Part model, mm, in its own coordinate system. Coordinates: 2 decimals unless noted, no trailing zeros. Loops run counter-clockwise (first coordinate to the right, second up) from the corner with the lowest first, then second, coordinate; pieces in that order, holes last. Notation, with made-up numbers: M 60,73 L 75,73 A6 ccw 75,79 Z; hole C 43.5,-20 d8. An arc over 180 degrees is marked long. Answer as CSV lines item,"result". Start each with the question number.
from build123d import *

# Parameters (mm, degrees)
F0_W     = 3.8
F0_H     = 1
F1_DEPTH = 2
F0_R     = 8.45
F0_W_2   = 24.8
F0_H_2   = 24.8
F2_DEPTH = 1
F3_R     = 2.7
F4_DEPTH = 0.5
F5_DEPTH = 1.5


with BuildPart() as f1:
    # F0 (on Top) → F1 (new body)
    with BuildSketch(Plane.XY):
        with Locations((21, 16.5)):
            Rectangle(F0_W, F0_H)
    extrude(amount=-F1_DEPTH)

    # F0 (on Top) → F2 (join)
    with BuildSketch(Plane.XY):
        with BuildLine():
            Line((19.1, 17), (0, 17))
            ThreePointArc((0, 17), (-17, 0), (0, -17))
            Line((0, -17), (53, -17))
            Line((53, -17), (53, -12.4))
            Line((53, -12.4), (28.2, -12.4))
            Line((28.2, -12.4), (28.2, 12.4))
            Line((28.2, 12.4), (53, 12.4))
            Line((53, 12.4), (53, 17))
            Line((53, 17), (22.9, 17))
            Line((22.9, 17), (22.9, 16))
            Line((22.9, 16), (19.1, 16))
            Line((19.1, 16), (19.1, 17))
        make_face()
        Circle(F0_R, mode=Mode.SUBTRACT)
        with Locations((21, 16.5)):
            Rectangle(F0_W, F0_H)
        with Locations((40.6, 0)):
            Rectangle(F0_W_2, F0_H_2)
    extrude(amount=-F2_DEPTH)

    # F3 (on face) → F4 (cut)
    with BuildSketch(Plane(origin=(0, 0, -1), x_dir=(1, 0, 0), z_dir=(0, 0, -1))):
        with Locations((19, 0)):
            Circle(F3_R)
    extrude(amount=-F4_DEPTH, mode=Mode.SUBTRACT)

    # F0 (on Top) → F5 (join)
    with BuildSketch(Plane.XY):
        with Locations((40.6, 0)):
            Rectangle(F0_W_2, F0_H_2)
    extrude(amount=-F5_DEPTH)


solid = f1.part
Q1. Slice it at A-A, the plane y = 0. Write the cut outline in (x, z), and give its area (3 significant figures).
Q2. Wall check: L1, parallel to Y at x = 19, z = -0.8; L2, parallel to Z at x = -6, y = -7; L3, parallel to Z at x = 42.5, y = -8.5. Give the ranges that are in metal, low to high.
Q3. Slice it at C-C, the plane x = -3.5. Write the cut outline in (y, z).
Q4. Slice it at B-B, the plane x = 47. Write the cut outline in (y, z), and give its area (3 significant figures).
Q5. Flat gauge pins, fed straight in: P1, Ø12.5, axis at x = 44, y = 0.5, coming from the -Z side; P2, Ø0.8, axis at y = 16.5, z = -1.5, coming from the -X side; P3, Ø5, axis at x = 19, y = 0, coming from the -Z side. Where does each tip first touch, or does it go through?
Q6. Slice it at D-D, the plane y = -10. Write the cut outline in (x, z).
Q7. Two-plate mould, pull along X, no slides. Class faces 1 (the face through (21.494, 1.034, -0.754)), 2 (the face through (40, 0, -1.5)), 3 (the face through (19, 0, -0.5)), 4 (the face through (-16.996, 0.374, -0.493)): +X half, -X half, draft (parallel to the pull), parting line (faces both ways), or undercut.
Solved:
1,outline,"M -17,-1 L -8.45,-1 L -8.45,0 L -17,0 Z; M 8.45,-1 L 16.3,-1 L 16.3,-0.5 L 21.7,-0.5 L 21.7,-1 L 28.2,-1 L 28.2,-1.5 L 53,-1.5 L 53,0 L 8.45,0 Z"
1,area,"62.8 mm2"
2,L1,"y = -17 to -2.7, 2.7 to 17"
2,L2,"z = -1 to 0"
2,L3,"z = -1.5 to 0"
3,outline,"M -16.64,-1 L -7.69,-1 L -7.69,0 L -16.64,0 Z; M 7.69,-1 L 16.64,-1 L 16.64,0 L 7.69,0 Z"
4,outline,"M -17,-1 L -12.4,-1 L -12.4,-1.5 L 12.4,-1.5 L 12.4,-1 L 17,-1 L 17,0 L -17,0 Z"
4,area,"46.4 mm2"
5,P1,"stops at z = -1.5"
5,P2,"stops at x = 19.1"
5,P3,"stops at z = -0.5"
6,outline,"M -13.75,-1 L 28.2,-1 L 28.2,-1.5 L 53,-1.5 L 53,0 L -13.75,0 Z"
7,face 1,"undercut"
7,face 2,"draft"
7,face 3,"undercut"
7,face 4,"-X half"
